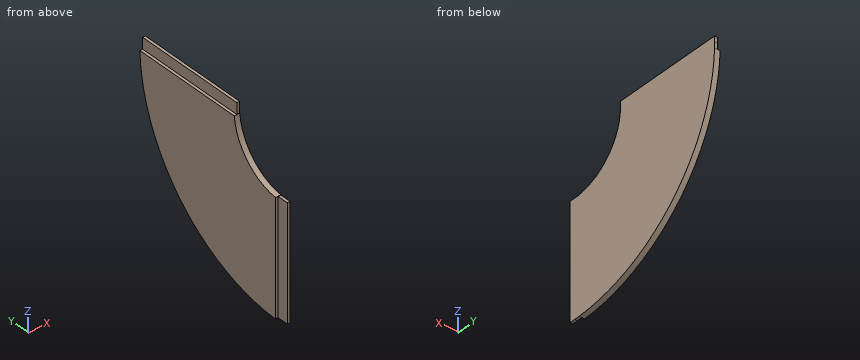
Autodesk Inventor part; units mm, degrees
ref_plane "YZ Plane" through (0, 0, 0) normal (1, 0, 0) x (0, 1, 0)
ref_plane "XZ Plane" through (0, 0, 0) normal (0, 1, 0) x (-1, 0, 0)
ref_plane "XY Plane" through (0, 0, 0) normal (0, 0, 1) x (1, 0, 0)
sketch "Sketch1" plane through (0, 0, 0) normal (1, 0, 0) x (0, 1, 0)
  line L0 (152.4, 0) -> (152.4, -152.4)
  line L1 (152.4, -152.4) -> (0, -152.4)
  circle A0 centre (0, 0) radius 152.4
  arc A1 (0, -152.4) -> (152.4, 0) centre (0, 0) ccw
  line L2 (152.318, 5) -> (50, 5)
  line L3 (50, -5) -> (50, 5)
  line L4 (152.318, -5) -> (49.7494, -5)
  line L5 (5, -49.7494) -> (5, -152.318)
  line L6 (-5, -50) -> (-5, -152.318)
  line L7 (5, -50) -> (-5, -50)
  arc A2 (50, 0) -> (0, -50) centre (0, 0) ccw
  arc A3 (5, -49.7494) -> (49.7494, -5) centre (0, 0) ccw
  dimension "d7" = 152.4
  dimension "d8" = 50
  dimension "d9" = 50
  dimension "d10" = 147.4
  dimension "d11" = 157.4
  dimension "d12" = 10
  dimension "d13" = 157.4
  dimension "d14" = 147.4
extrude "Extrusion1" add sketch "Sketch1" along normal blind 5 contours A0 L5 A3 L4
sketch "Sketch2" plane through (5, 0, 0) normal (1, 0, 0) x (0, 0, -1)
  line L0 (49.7494, 5) -> (152.318, 5)
  line L1 (50, 5) -> (50, -5)
  line L2 (0, 152.4) -> (0, 0)
  line L3 (5, 152.318) -> (5, 49.7494)
  line L4 (0, 0) -> (152.4, 0)
  arc A0 (152.4, 0) -> (0, 152.4) centre (0, 0) ccw
  arc A1 (152.318, 5) -> (5, 152.318) centre (0, 0) ccw
  line L5 (50, -5) -> (152.318, -5)
  arc A2 (152.318, -5) -> (152.318, 5) centre (0, 0) ccw
  line L6 (-5, 50) -> (5, 50)
  line L7 (5, 50) -> (5, 152.318)
  arc A3 (5, 152.318) -> (-5, 152.318) centre (0, 0) ccw
  line L8 (-5, 152.318) -> (-5, 50)
  arc A4 (49.7494, 5) -> (5, 49.7494) centre (0, 0) ccw
  arc A5 (0, 50) -> (50, 0) centre (0, 0) ccw
  point P0 (0, 152.4)
  dimension "d18" = 10
  dimension "d19" = 152.4
  dimension "d20" = 152.4
  dimension "d23" = 90
  dimension "d25" = 152.4
extrude "Extrusion2" add sketch "Sketch2" against normal blind 2.5 contours L0 A0 L4 L1 | L4 A2 L5 L1 | L6 L2 A0 L3 | L6 L8 A3 L2
Read the model definition and answer for the solid it produces. Units are mm, in the model's axes. Give positions to 0.01 mm unless a question says otherwise; leave off trailing zeros. Write each loop counter-clockwise with the first axis right and the second up, starting at its lowest first coordinate (ties: lowest second). Pieces come first, ordered by that corner, then holes. Notation, with made-up numbers: (5, 70) - (56, 70) arc R10 ccw to (56, 80) - close; hole circle Ø4 at (66.25, -19.75). An arc over 180 degrees is marked (long way). Use CSV: the item, a comma, the result in double quotes. Start each with the question number.
(1) Consider line 1 along Z through (x, y) = (3.9, 2.5); line 2 along Y through (x, z) = (0.65, -58); line 3 along Z through (x, y) = (2.7, 133). Determine where each line is inside the solid, lowest interval first.
(2) Find section A-A (y = 115.5). Give the vertices of the cut face in (x, z).
(3) Given P1, Ø1.2, axis at x = 4, z = -1.5, coming from the -Y side; P2, Ø8, axis at y = -1.5, z = -87, coming from the -X side; P3, Ø10, axis at y = 108, z = -115.5, coming from the +X side; P4, Ø2, axis at x = 1.5, y = 40, coming from the +Z side, each flat-ended and moving along its own axis, determine where each tip first touches the part or whether it passes through.
(4) Find section B-B (z = -76.5). Give the vertices of the cut face in (x, y), plus the area to 3 significant figures.
(5) Find section D-D (y = 38). Give the vertices of the cut face in (x, z), plus the area to 3 significant figures.
(6) Find section C-C (x = 1.35). Give the vertices of the cut face in (y, z).
Findings below:
1,line 1,"-152.38 to -50"
1,line 2,"5 to 140.93"
1,line 3,"-74.41 to 5"
2,outline,"(0, -99.43) - (5, -99.43) - (5, 5) - (2.5, 5) - (2.5, -5) - (0, -5) - close"
3,P1,"y = 50"
3,P2,"x = 2.5"
3,P3,"through"
3,P4,"z = -28.62"
4,outline,"(0, 5) - (2.5, 5) - (2.5, -5) - (5, -5) - (5, 131.81) - (0, 131.81) - close"
4,area,"659 mm2"
5,outline,"(0, -147.59) - (5, -147.59) - (5, -32.5) - (0, -32.5) - close"
5,area,"575 mm2"
6,outline,"(5, -152.32) arc R152.4 ccw to (152.32, -5) - (49.75, -5) arc R50 cw to (5, -49.75) - close"
